Geometry check sheet. Reference: drawing and pictorial views, mm from the part's lowest x, y, z. A direction names the side the tool comes from. Give positions to 0.01 mm unless a question says otherwise; leave off trailing zeros. Loops run counter-clockwise (first coordinate to the right, second up) from the corner with the lowest first, then second, coordinate; pieces in that order, holes last. Notation, with made-up numbers: (22.5, -9.5) - (65.5, -9.5) arc R10 ccw to (65.5, 1.5) - close; hole circle Ø3 at (-4, -5.75). An arc over 180 degrees is marked (long way). Answer in a Markdown table with one row per item. Add a question column.
(1) Thickness scan on L1, parallel to X at y = 6.8, z = 11.5; L2, parallel to X at y = 8.25, z = 11.5; L3, parallel to Z at x = 11.5, y = 1.3. Record the ranges inside material, lowest first.
(2) Sectioned sample at A-A on x = 11.5. Enter the section's corners in (y, z).
(3) Go/stop test with flat-tipped pins: P1, Ø6, axis at y = 1.5, z = 5, coming from the -X side (1 decimal); P2, Ø4.5, axis at x = 12, z = 11.5, coming from the +Y side; P3, Ø5, axis at x = 13, z = 11, coming from the +Y side. Record where each tip stops, or that it passes through.
(4) Set-up check for the marked faces 1 and 2: record each of +Z, -Z, +X, -X, +Y, -Y from which the full face is reachable in a straight line by a thin tool's end or side.
(5) Sectioned sample at D-D on y = 2.5. Enter the section's corners in (x, z), then the cut area to 3 significant figures.
(6) Sectioned sample at C-C on y = 7.75. Enter the section's corners in (x, z) (1 decimal), then the cut area to 3 significant figures.
(7) Draft check along X on the marked faces 3, 4 and 5. Enter one of: released by +X, released by -X, zero draft, split by the parting line, or undercut.
(8) Sectioned sample at B-B on z = 11.5. Enter the section's corners in (x, y).
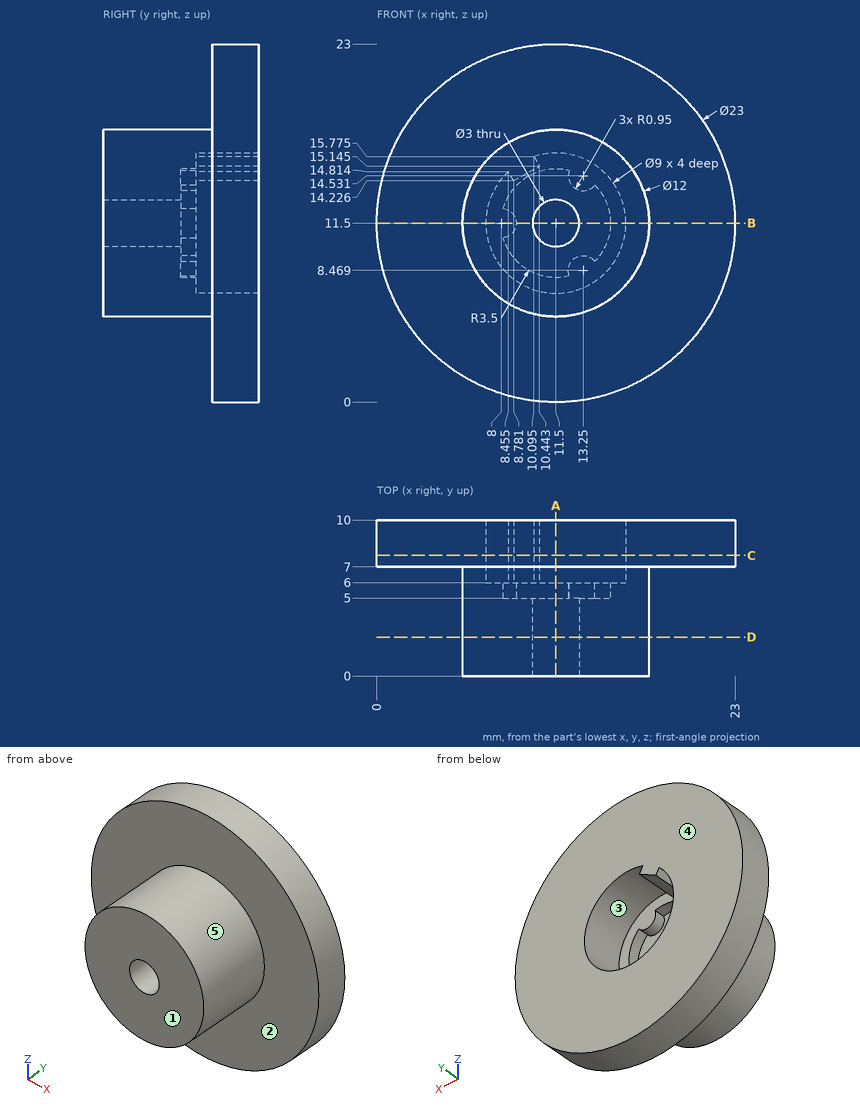
Reply:
| question | item | result |
|---|---|---|
| 1 | L1 | 5.5 to 7, 16 to 17.5 |
| 1 | L2 | 0 to 7, 16 to 23 |
| 1 | L3 | 5.5 to 10, 13 to 17.5 |
| 2 | outline | (0, 5.5) - (7, 5.5) - (7, 0) - (10, 0) - (10, 7) - (6, 7) - (6, 8) - (5, 8) - (5, 10) - (0, 10) - close; (0, 13) - (5, 13) - (5, 15) - (6, 15) - (6, 16) - (10, 16) - (10, 23) - (7, 23) - (7, 17.5) - (0, 17.5) - close |
| 3 | P1 | x = 6.6 |
| 3 | P2 | y = 5 |
| 3 | P3 | y = 6 |
| 4 | face 1 | +Z, -Z, +X, -X, -Y |
| 4 | face 2 | -Y |
| 5 | outline | circle Ø12 at (11.5, 11.5); hole circle Ø3 at (11.5, 11.5) |
| 5 | area | 106 mm^2 |
| 6 | outline | circle Ø23 at (11.5, 11.5); hole (8.5, 14.8) arc R4.5 ccw (long way) to (10.1, 15.8) - (10.4, 15.1) - (8.8, 14.2) - close |
| 6 | area | 353 mm^2 |
| 7 | face 3 | undercut |
| 7 | face 4 | zero draft |
| 7 | face 5 | split by the parting line |
| 8 | outline | (0, 7) - (5.5, 7) - (5.5, 0) - (10, 0) - (10, 5) - (8.95, 5) - (8.95, 6) - (7, 6) - (7, 10) - (0, 10) - close; (13, 0) - (17.5, 0) - (17.5, 7) - (23, 7) - (23, 10) - (16, 10) - (16, 6) - (15, 6) - (15, 5) - (13, 5) - close |
